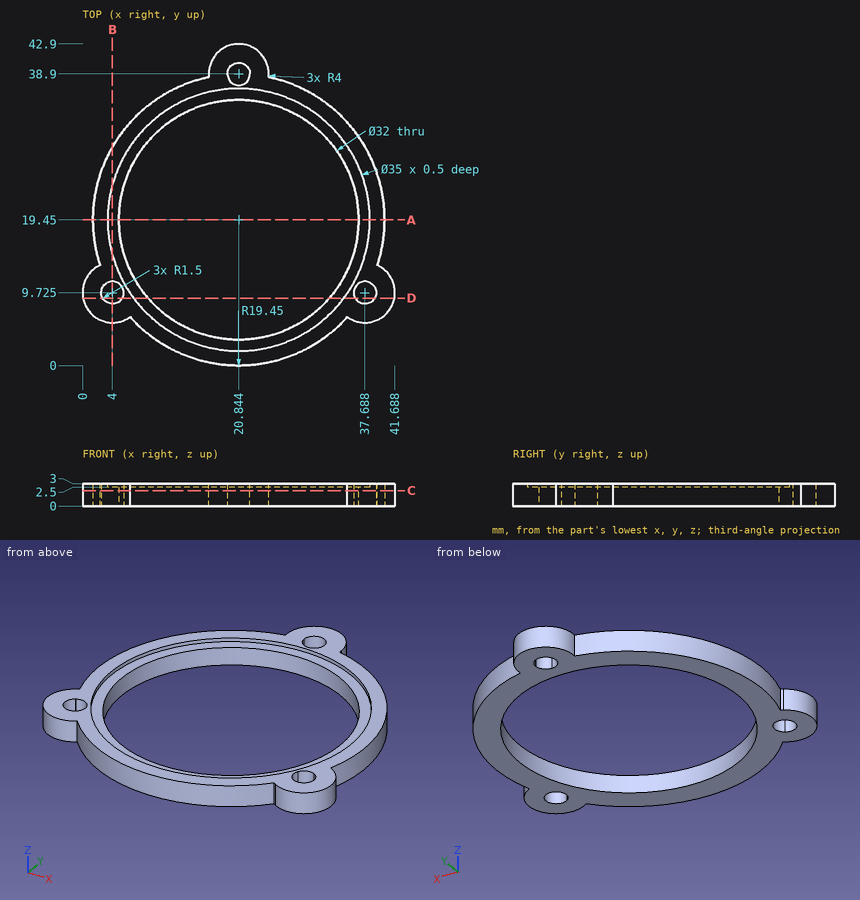
Here's the drawing with two shaded views (mm, measured from the low corner). I have some questions. Round coordinates to 2 decimals unless told otherwise and drop trailing zeros. Order: outer loops, then holes, each group sorted by start corner. A loop starts at its lowest first (then second) coordinate and runs counter-clockwise, first axis right, second up. Notation, with made-up numbers: (6, 83) -> (16, 83) arc R11 ccw to (16, 100) -> close; hole circle Ø8 at (58, 68.5). An arc over 180 degrees is marked (long way). Write each question's results on one line, items separated by ' | '. Start each with the question number.
Item 1: Will these pins go through, and if not, where does the flat tip stop? pin 1 (1 mm diameter, centred on x = 18.5, z = 2, fed in from +Y); pin 2 (1.5 mm diameter, centred on x = 34.5, z = 2.5, fed in from -Y).
Item 2: If we section it at B-B, the plane x = 4: Write out the boundary of the cut face in (y, z) (1 decimal).
Item 3: Please list where these lines run through material, in increasing order: L1, parallel to X at y = 20, z = 1.6 (1 decimal); L2, parallel to Y at x = 21, z = 1.3; L3, parallel to X at y = 19.5, z = 0.7 (1 decimal).
Item 4: If we section it at A-A, the plane y = 19.45: Write out the boundary of the cut face in (x, z).
Item 5: If we section it at D-D, the plane y = 9: Write out the boundary of the cut face in (x, z) (1 decimal), then the cut area to 3 significant figures.
Item 6: If we section it at C-C, the plane z = 2.05: State how many separate pieces and enclosed holes the cut face has, then the cut area to 3 significant figures.
Results:
1) pin 1: stops at y = 42.45 | pin 2: stops at y = 4.9
2) outline: (5.7, 0) -> (8.2, 0) -> (8.2, 3) -> (5.7, 3) -> close; (11.2, 0) -> (29.2, 0) -> (29.2, 3) -> (24.2, 3) -> (24.2, 2.5) -> (14.7, 2.5) -> (14.7, 3) -> (11.2, 3) -> close
3) L1: x = 1.4 to 4.9, 36.8 to 40.3 | L2: y = 0 to 3.45, 35.45 to 37.41, 40.39 to 42.9 | L3: x = 1.4 to 4.8, 36.8 to 40.3
4) outline: (1.39, 0) -> (4.84, 0) -> (4.84, 2.5) -> (3.34, 2.5) -> (3.34, 3) -> (1.39, 3) -> close; (36.84, 0) -> (40.29, 0) -> (40.29, 3) -> (38.34, 3) -> (38.34, 2.5) -> (36.84, 2.5) -> close
5) outline: (0.1, 0) -> (2.7, 0) -> (2.7, 3) -> (0.1, 3) -> close; (5.3, 0) -> (8.7, 0) -> (8.7, 2.5) -> (6.8, 2.5) -> (6.8, 3) -> (5.3, 3) -> close; (33, 0) -> (36.4, 0) -> (36.4, 3) -> (34.9, 3) -> (34.9, 2.5) -> (33, 2.5) -> close; (39, 0) -> (41.6, 0) -> (41.6, 3) -> (39, 3) -> close | area: 34.3 mm2
6) separate pieces: 1 | enclosed holes: 4 | area: 442 mm2
